The figure shows three views and two pictorial views of one solid part (mm, origin at its lowest corner). Answer the questions. Round coordinates to 2 decimals unless told otherwise and drop trailing zeros. Loops run counter-clockwise (first coordinate to the right, second up) from the corner with the lowest first, then second, coordinate; pieces in that order, holes last. Notation, with made-up numbers: (68.5, 7.5) -> (113.5, 7.5) arc R21 ccw to (113.5, 13.5) -> close; hole circle Ø11 at (16.5, -39). An arc over 180 degrees is marked (long way). Use a Markdown table: item, result. Add a question column.
Q1. Consider line 1 (X direction, y = 0.8, z = 27.5); line 2 (Z direction, x = 8.5, y = 0.75). Determine where each line is inside the solid, lowest interval first.
Q2. Section C-C on y = 0.5 is taken. Give the vertices of the cut face in (x, z).
Q3. Section A-A on x = 7.5 is taken. Give the vertices of the cut face in (y, z), then the cut area to 3 significant figures.
Q4. Section D-D on z = 7.5 is taken. Give the vertices of the cut face in (x, y), then the cut area to 3 significant figures.
Q5. Given pin 1 Ø2.5 at (x, z) = (7.5, 17.5) entering from +Y, flat-ended and moving along its own axis, determine where the tip first touches the part or whether it passes through.
Q6. Section B-B on z = 27.5 is taken. Give the vertices of the cut face in (x, y).
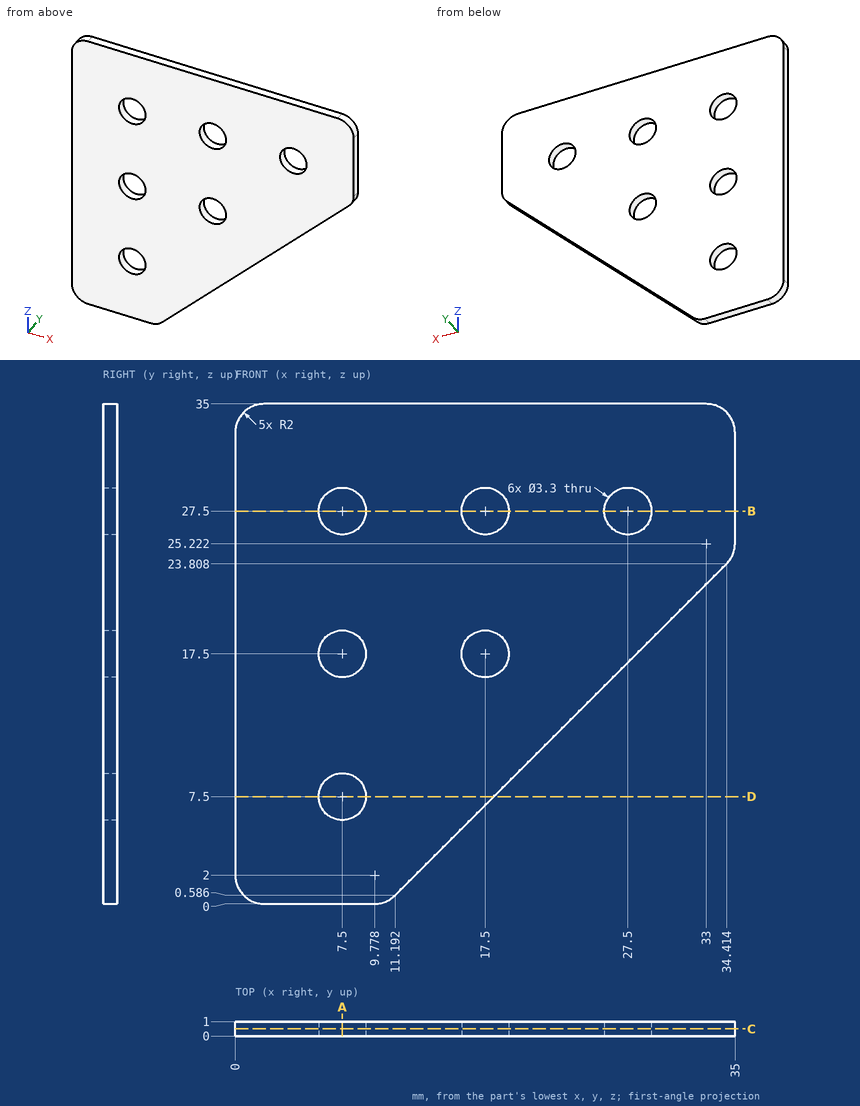
Checked values:
| question | item | result |
|---|---|---|
| 1 | line 1 | x = 0 to 5.85, 9.15 to 15.85, 19.15 to 25.85, 29.15 to 35 |
| 1 | line 2 | z = 0 to 6.19, 8.81 to 16.19, 18.81 to 26.19, 28.81 to 35 |
| 2 | outline | (0, 2) arc R2 ccw to (2, 0) -> (9.78, 0) arc R2 ccw to (11.19, 0.59) -> (34.41, 23.81) arc R2 ccw to (35, 25.22) -> (35, 33) arc R2 ccw to (33, 35) -> (2, 35) arc R2 ccw to (0, 33) -> close; hole circle Ø3.3 at (7.5, 7.5); hole circle Ø3.3 at (7.5, 17.5); hole circle Ø3.3 at (7.5, 27.5); hole circle Ø3.3 at (17.5, 17.5); hole circle Ø3.3 at (17.5, 27.5); hole circle Ø3.3 at (27.5, 27.5) |
| 3 | outline | (0, 0) -> (1, 0) -> (1, 5.85) -> (0, 5.85) -> close; (0, 9.15) -> (1, 9.15) -> (1, 15.85) -> (0, 15.85) -> close; (0, 19.15) -> (1, 19.15) -> (1, 25.85) -> (0, 25.85) -> close; (0, 29.15) -> (1, 29.15) -> (1, 35) -> (0, 35) -> close |
| 3 | area | 25.1 mm2 |
| 4 | outline | (0, 0) -> (5.85, 0) -> (5.85, 1) -> (0, 1) -> close; (9.15, 0) -> (18.11, 0) -> (18.11, 1) -> (9.15, 1) -> close |
| 4 | area | 14.8 mm2 |
| 5 | pin 1 | passes through |
| 6 | outline | (0, 0) -> (5.85, 0) -> (5.85, 1) -> (0, 1) -> close; (9.15, 0) -> (15.85, 0) -> (15.85, 1) -> (9.15, 1) -> close; (19.15, 0) -> (25.85, 0) -> (25.85, 1) -> (19.15, 1) -> close; (29.15, 0) -> (35, 0) -> (35, 1) -> (29.15, 1) -> close |
